Read the model definition and answer for the solid it produces. Units are mm, in the model's axes. Face numbers are marked on the shaded views. A direction names the side the tool comes from. Give positions to 0.01 mm unless a question says otherwise; leave off trailing zeros. Write each loop counter-clockwise with the first axis right and the second up, starting at its lowest first coordinate (ties: lowest second). Pieces come first, ordered by that corner, then holes. Notation, with made-up numbers: M 16.25,-27 L 73.25,-27 A32 ccw 73.25,9 Z; hole C 29.25,-20.75 d10. An arc over 180 degrees is marked long. Use a Markdown table: item, result. Add a question column.
Item 1: A cutting plane is placed at A-A on x = 0. Determine the outline of the cut face in (y, z) (3 decimals), then the cut area to 3 significant figures.
Item 2: Given P1, Ø2, axis at x = -5.08, z = 0, coming from the -Y side; P2, Ø5, axis at x = 6, y = 25.5, coming from the -Z side; P3, Ø4, axis at x = 3, y = 6.5, coming from the -Z side, each flat-ended and moving along its own axis, determine where each tip first touches the part or whether it passes through.
Item 3: For the marked faces 4, 5 and 6, determine the directions among +Z, -Z, +X, -X, +Y, -Y from which every point of the face is accessible in a straight line to the end or side of a thin tool.
Item 4: A cutting plane is placed at D-D on z = -0.75. Determine the outline of the cut face in (x, y), then the cut area to 3 significant figures.
Item 5: The mould has two halves that part along X. Classify the marked faces 1, 2 and 3: pulls with the +X half, pulls with the -X half, needs draft (parallel to the pull), parting line crosses it, or undercut.
Item 6: A cutting plane is placed at B-B on z = 3. Determine the outline of the cut face in (x, y), then the cut area to 3 significant figures.
Item 7: A cutting plane is placed at C-C on y = 20. Determine the outline of the cut face in (x, z).
Item 8: Consider probe 1 along X at (y, z) = (3.25, 0); probe 2 along Y at (x, z) = (1.25, -6); probe 3 along Y at (x, z) = (-5.5, 0). Determine where each line is inside the solid, lowest interval first. Write a range as [from, to].
from build123d import *

# Parameters (mm, degrees)
SKETCH1_R           = 7.62
BOSS_EXTRUDE1_DEPTH = 29.8196
SKETCH2_R           = 3.975
BOSS_EXTRUDE2_DEPTH = 7.62
SKETCH3_R           = 1.1938
CUT_EXTRUDE1_DEPTH  = 7.8232


with BuildPart() as part:
    # Sketch1 → Boss-Extrude1 (new body)
    with BuildSketch(Plane(origin=(0, 0, 0), x_dir=(1, 0, 0), z_dir=(0, 1, 0))):
        with Locations(Location((0, 0, 0), (0, 0, 270))):
            Circle(SKETCH1_R)
    extrude(amount=BOSS_EXTRUDE1_DEPTH)

    # Sketch2 → Boss-Extrude2 (add)
    with BuildSketch(Plane(origin=(0, 29.8196, 0), x_dir=(1, 0, 0), z_dir=(0, 1, 0))):
        with Locations(Location((0, 0, 0), (0, 0, 90))):
            Circle(SKETCH2_R)
    extrude(amount=BOSS_EXTRUDE2_DEPTH)

    # Sketch3 → Cut-Extrude1 (cut)
    with BuildSketch(Plane.XZ):
        with Locations(Location((-5.08, 0, 0), (0, 0, 270))):
            Circle(SKETCH3_R)
        with Locations(Location((5.08, 0, 0), (0, 0, 270))):
            Circle(SKETCH3_R)
    extrude(amount=-CUT_EXTRUDE1_DEPTH, mode=Mode.SUBTRACT)


solid = part.part
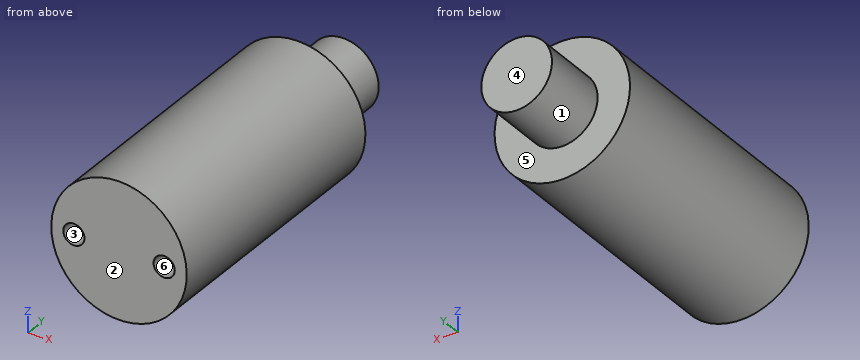
Filled in:
| question | item | result |
|---|---|---|
| 1 | outline | M 0,-7.62 L 29.82,-7.62 L 29.82,-3.975 L 37.44,-3.975 L 37.44,3.975 L 29.82,3.975 L 29.82,7.62 L 0,7.62 Z |
| 1 | area | 515 mm² |
| 2 | P1 | y = 7.82 |
| 2 | P2 | z = -6.77 |
| 2 | P3 | z = -7.55 |
| 3 | face 4 | +Z, -Z, +X, -X, +Y |
| 3 | face 5 | +Y |
| 3 | face 6 | -Y |
| 4 | outline | M -7.58,0 L -6.01,0 L -6.01,7.82 L -4.15,7.82 L -4.15,0 L 4.15,0 L 4.15,7.82 L 6.01,7.82 L 6.01,0 L 7.58,0 L 7.58,29.82 L 3.9,29.82 L 3.9,37.44 L -3.9,37.44 L -3.9,29.82 L -7.58,29.82 Z |
| 4 | area | 483 mm² |
| 5 | face 1 | parting line crosses it |
| 5 | face 2 | needs draft |
| 5 | face 3 | undercut |
| 6 | outline | M -7,0 L 7,0 L 7,29.82 L 2.61,29.82 L 2.61,37.44 L -2.61,37.44 L -2.61,29.82 L -7,29.82 Z |
| 6 | area | 457 mm² |
| 7 | outline | C 0,0 d15.24 |
| 8 | probe 1 | [-7.62, -6.27], [-3.89, 3.89], [6.27, 7.62] |
| 8 | probe 2 | [0, 29.82] |
| 8 | probe 3 | [7.82, 29.82] |
